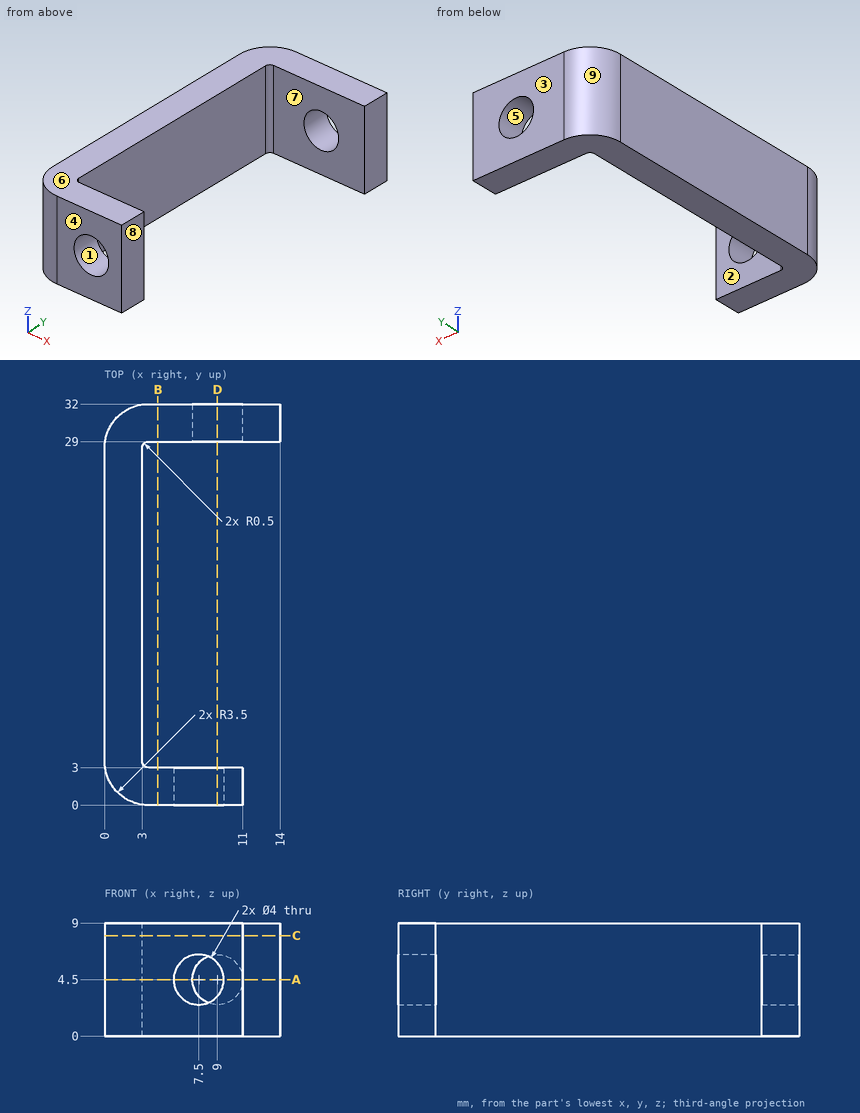
Study the drawing (mm; zero at the part's minimum x, y, z) and answer. A direction names the side the tool comes from. Round coordinates to 2 decimals unless told otherwise and drop trailing zeros. Write each loop counter-clockwise with the first axis right and the second up, starting at its lowest first coordinate (ties: lowest second). Pieces come first, ordered by that corner, then holes. Notation, with made-up numbers: (-3.75, 12.25) - (6.25, 12.25) arc R26 ccw to (6.25, 37.25) - close; hole circle Ø8 at (78.5, 83.25). An arc over 180 degrees is marked (long way). Return JSON: item names as keys, results as strings. Group by question number.
Q1. The part is cut by section C-C on z = 8. Write down the section's boundary in (x, y), then the cut area to 3 significant figures.
Q2. Find the intervals of material crossed by L1, parallel to Z at x = 9, y = 30.8; L2, parallel to Y at x = 9.25, z = 7.5; L3, parallel to X at y = 6, z = 2, in increasing order.
Q3. The part is cut by section A-A on z = 4.5. Write down the section's boundary in (x, y).
Q4. The mould has two halves that part along Y. Classify the marked faces 1, 2, 3 and 4: released by +Y, released by -Y, zero draft, split by the parting line, or undercut.
Q5. Each of these flat-tipped pins is pushed along its axis until it touches: pin 1 Ø5 at (x, y) = (7, 10.5) entering from -Z; pin 2 Ø3 at (x, z) = (7.5, 4.5) entering from -Y; pin 3 Ø3.5 at (y, z) = (2, 6.5) entering from +X. Where does it stop, or does it pass through?
Q6. The part is cut by section B-B on x = 4.25. Write down the section's boundary in (y, z).
Q7. The part is cut by section D-D on x = 9. Write down the section's boundary in (y, z).
Q8. For the marked faces 5, 6, 7, 8 and 9, determine the directions among +Z, -Z, +X, -X, +Y, -Y from which every point of the face is accessible in a straight line to the end or side of a thin tool.
Solved:
{
 "1": {"outline": "(0, 3.5) arc R3.5 ccw to (3.5, 0) - (11, 0) - (11, 3) - (3.5, 3) arc R0.5 cw to (3, 3.5) - (3, 28.5) arc R0.5 cw to (3.5, 29) - (14, 29) - (14, 32) - (3.5, 32) arc R3.5 ccw to (0, 28.5) - close", "area": "148 mm²"},
 "2": {"L1": "0 to 2.5, 6.5 to 9", "L2": "0 to 3, 29 to 32", "L3": "0 to 3"},
 "3": {"outline": "(0, 3.5) arc R3.5 ccw to (3.5, 0) - (5.5, 0) - (5.5, 3) - (3.5, 3) arc R0.5 cw to (3, 3.5) - (3, 28.5) arc R0.5 cw to (3.5, 29) - (7, 29) - (7, 32) - (3.5, 32) arc R3.5 ccw to (0, 28.5) - close; (9.5, 0) - (11, 0) - (11, 3) - (9.5, 3) - close; (11, 29) - (14, 29) - (14, 32) - (11, 32) - close"},
 "4": {"face 1": "zero draft", "face 2": "undercut", "face 3": "released by +Y", "face 4": "released by -Y"},
 "5": {"pin 1": "through", "pin 2": "y = 29", "pin 3": "x = 11"},
 "6": {"outline": "(0, 0) - (3, 0) - (3, 9) - (0, 9) - close; (29, 0) - (32, 0) - (32, 9) - (29, 9) - close"},
 "7": {"outline": "(0, 0) - (3, 0) - (3, 3.18) - (0, 3.18) - close; (0, 5.82) - (3, 5.82) - (3, 9) - (0, 9) - close; (29, 0) - (32, 0) - (32, 2.5) - (29, 2.5) - close; (29, 6.5) - (32, 6.5) - (32, 9) - (29, 9) - close"},
 "8": {"face 5": "+Y", "face 6": "+Z, +X, -X, +Y, -Y", "face 7": "+Z, -Z, +X", "face 8": "+Z, -Z, +X, -Y", "face 9": "+Z, -Z, -X, +Y"}
}
